Can you work these out from the model? Positions are in its coordinate system, mm. Coordinates: 2 decimals unless noted, no trailing zeros. Loops run counter-clockwise (first coordinate to the right, second up) from the corner with the lowest first, then second, coordinate; pieces in that order, holes last.
```python
from build123d import *

# Parameters (mm, degrees)
SKETCH_1_R          = 5.2
SKETCH_1_R_2        = 9.7
EXTRUDE_1_DEPTH     = 4
SKETCH_2_R          = 2
CUT_EXTRUDE_1_DEPTH = 10
SKETCH_3_R          = 5
CUT_EXTRUDE_2_DEPTH = 10
SKETCH_4_R          = 1
CUT_EXTRUDE_3_DEPTH = 10


with BuildPart() as part:
    # 草图1 → 凸台-拉伸1 (new body)
    with BuildSketch(Plane.XY):
        with BuildLine():
            Line((250, 19.7), (0, 19.7))
            Line((0, 19.7), (-45, 15.2))
            ThreePointArc((-45, 15.2), (-60.2, 0), (-45, -15.2))
            Line((-45, -15.2), (0, -19.7))
            Line((0, -19.7), (250, -19.7))
            ThreePointArc((250, -19.7), (269.7, 0), (250, 19.7))
        make_face()
        Circle(SKETCH_1_R, mode=Mode.SUBTRACT)
        with Locations((250, 0)):
            Circle(SKETCH_1_R_2, mode=Mode.SUBTRACT)
        with Locations((-45, 0)):
            Circle(SKETCH_1_R, mode=Mode.SUBTRACT)
    extrude(amount=EXTRUDE_1_DEPTH)

    # 草图2 → 切除-拉伸1 (cut)
    with BuildSketch(Plane.XY.offset(4)):
        with Locations((25, 15)):
            Circle(SKETCH_2_R)
        with Locations((90, 15)):
            Circle(SKETCH_2_R)
        with Locations((155, 15)):
            Circle(SKETCH_2_R)
        with Locations((220, 15)):
            Circle(SKETCH_2_R)
        with Locations((90, -15)):
            Circle(SKETCH_2_R)
        with Locations((155, -15)):
            Circle(SKETCH_2_R)
        with Locations((220, -15)):
            Circle(SKETCH_2_R)
        with Locations((25, -15)):
            Circle(SKETCH_2_R)
    extrude(amount=-CUT_EXTRUDE_1_DEPTH, mode=Mode.SUBTRACT)

    # 草图3 → 切除-拉伸2 (cut)
    with BuildSketch(Plane.XY.offset(4)):
        with Locations((-22.5, 0)):
            Circle(SKETCH_3_R)
        with BuildLine():
            Line((32, 8), (32, -8))
            Line((32, -8), (88.462542093, -8))
            Line((88.462542093, -8), (114.86138476, 4.184081231))
            ThreePointArc((114.86138476, 4.184081231), (115.976706085, 6.429046887), (114.023268405, 8))
            Line((114.023268405, 8), (32, 8))
        make_face()
        with BuildLine():
            Line((156.537457907, 8), (213, 8))
            Line((213, 8), (213, -8))
            Line((213, -8), (130.976731595, -8))
            ThreePointArc((130.976731595, -8), (129.023293915, -6.429046887), (130.13861524, -4.184081231))
            Line((130.13861524, -4.184081231), (156.537457907, 8))
        make_face()
    extrude(amount=-CUT_EXTRUDE_2_DEPTH, mode=Mode.SUBTRACT)

    # 草图4 → 切除-拉伸3 (cut)
    with BuildSketch(Plane.XY.offset(4)):
        with Locations((250, 9.7)):
            Circle(SKETCH_4_R)
    extrude(amount=-CUT_EXTRUDE_3_DEPTH, mode=Mode.SUBTRACT)


solid = part.part
```
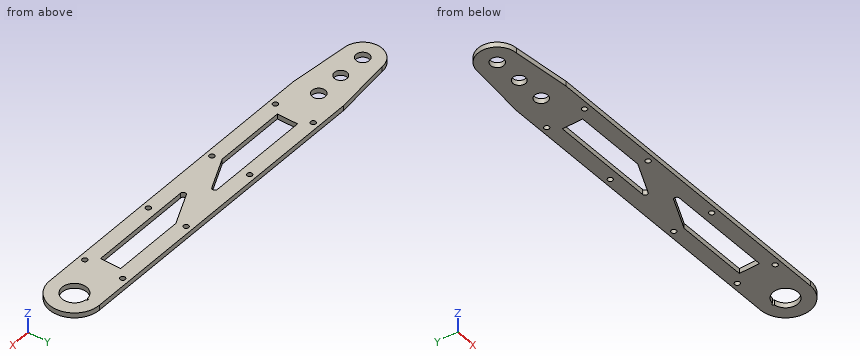
Item 1: I'm going to push flat-ended pins straight in: P1, Ø1, axis at y = 4, z = 1.5, coming from the -X side; P2, Ø2, axis at y = 1.5, z = 3, coming from the +X side. Where does each tip first touch, or does it pass through?
Results are:
P1: stops at x = -59.79
P2: stops at x = 269.69
Item 2: I need wall thicknesses on line 1 along Y through (x, z) = (220, 1.95); line 2 along Y through (x, z) = (220.5, 2.05); line 3 along Y through (x, z) = (56, 1.4). Which ranges of each line are inside material? Lowest first, please.
Results are:
line 1: y = -19.7 to -17, -13 to 13, 17 to 19.7
line 2: y = -19.7 to -16.94, -13.06 to 13.06, 16.94 to 19.7
line 3: y = -19.7 to -8, 8 to 19.7
Item 3: Suppose I cut it at C-C, the plane z = 2.3. Count the separate pieces of the cut face and the enclosed holes in it, plus the area to 3 significant figures.
Results are:
separate pieces: 1
enclosed holes: 14
area: 9,410 mm2
Item 4: Suppose I cut it at B-B, the plane y = 0. Please give me the cut outline in (x, z), plus the area to 3 significant figures.
Results are:
outline: (-60.2, 0) - (-50.2, 0) - (-50.2, 4) - (-60.2, 4) - close; (-39.8, 0) - (-27.5, 0) - (-27.5, 4) - (-39.8, 4) - close; (-17.5, 0) - (-5.2, 0) - (-5.2, 4) - (-17.5, 4) - close; (5.2, 0) - (32, 0) - (32, 4) - (5.2, 4) - close; (105.8, 0) - (139.2, 0) - (139.2, 4) - (105.8, 4) - close; (213, 0) - (240.3, 0) - (240.3, 4) - (213, 4) - close; (259.7, 0) - (269.7, 0) - (269.7, 4) - (259.7, 4) - close
area: 528 mm2
Item 5: Suppose I cut it at A-A, the plane x = -22.5. Please give me the cut outline in (y, z), plus the area to 3 significant figures.
Results are:
outline: (-17.45, 0) - (-5, 0) - (-5, 4) - (-17.45, 4) - close; (5, 0) - (17.45, 0) - (17.45, 4) - (5, 4) - close
area: 99.6 mm2
